Autodesk Inventor part; units mm, degrees
ref_plane "YZ Plane" through (0, 0, 0) normal (1, 0, 0) x (0, 1, 0)
ref_plane "XZ Plane" through (0, 0, 0) normal (0, 1, 0) x (-1, 0, 0)
ref_plane "XY Plane" through (0, 0, 0) normal (0, 0, 1) x (1, 0, 0)
sketch "Sketch1" plane through (0, 0, 0) normal (0, 1, 0) x (-1, 0, 0)
  line L0 (-10, 11.5) -> (10, 11.5)
  line L1 (10, 11.5) -> (10, -11.5)
  line L2 (10, -11.5) -> (-10, -11.5)
  line L3 (-10, -11.5) -> (-10, 11.5)
  line L4 (-10, 11.5) -> (10, -11.5) construction
  line L5 (10, 11.5) -> (-10, -11.5) construction
  point P0 (0, 0)
  dimension "d0" = 20
  dimension "d1" = 23
extrude "Extrusion2" add sketch "Sketch1" against normal blind 20
ref_plane "Work Plane1" through (-10, 0, 0) normal (0, 0, 1) x (1, 0, 0)
ref_plane "Work Plane2" through (0, -2, 0) normal (0, 1, 0) x (1, 0, 0)
sketch "Sketch11" plane through (0, -2, 0) normal (0, 1, 0) x (1, 0, 0)
  point P0 (0, 0)
sketch "Sketch12" plane through (10, 0, 11.5) normal (1, 0, 0) x (0, 0, -1)
  line L0 (23, -20) -> (0, -20)
  line L1 (0, -20) -> (0, 0)
  line L2 (0, 0) -> (23, 0)
  line L3 (23, 0) -> (23, -20)
  point P0 (11.5, 0)
  dimension "d41" = 23
  dimension "d42" = 20
extrude "Extrusion4" add sketch "Sketch12" along normal blind 22
sketch "Sketch13" plane through (32, 0, 11.5) normal (1, 0, 0) x (0, 0, -1)
  line L0 (23, 0) -> (23, -20)
  line L1 (23, -20) -> (3, -20)
  line L2 (3, -20) -> (3, 0)
  line L3 (3, 0) -> (23, 0)
  line L4 (23, 0) -> (23, -20)
  point P0 (11.5, 0)
  dimension "d45" = 20
extrude "Extrusion5" add sketch "Sketch13" along normal blind 120
sketch "Sketch26" plane through (32, -20, 8.5) normal (0, 0, 1) x (1, 0, 0)
  line L0 (8, 15) -> (23, 15)
  line L1 (23, 15) -> (23, 5)
  line L2 (23, 5) -> (8, 5)
  line L3 (8, 5) -> (8, 15)
  line L4 (0, 20) -> (120, 20)
  line L5 (0, 0) -> (120, 0)
  point P0 (-32, 20)
  dimension "d91" = 15
  dimension "d92" = 10
  dimension "d93" = 5
  dimension "d94" = 5
extrude "Extrusion12" cut sketch "Sketch26" against normal blind 15
sketch "Sketch28" plane through (10, 0, -11.5) normal (0, 0, -1) x (-1, 0, 0)
  line L0 (-22, 0) -> (-22, -20)
  line L1 (20, -20) -> (-142, -20)
  line L2 (-22, 0) -> (-142, 0)
  point P0 (10, 0)
  point P1 (-27, -17)
  point P2 (-46, -3)
  dimension "d101" = 19
  dimension "d102" = 5
  dimension "d103" = 3
  dimension "d104" = 3
hole "Hole3" at (56, -3, -11.5) at (37, -17, -11.5) direction (0, 0, 1) diameter 3.5 end through all counterbore diameter 5.5 counterbore depth 4
sketch "Sketch29" plane through (0, -20, 0) normal (0, -1, 0) x (1, 0, 0)
  line L0 (10, 11.5) -> (-10, 11.5)
  line L1 (10, -11.5) -> (10, 11.5)
  line L2 (-10, -11.5) -> (152, -11.5)
  line L3 (-10, 11.5) -> (-10, -11.5)
  point P0 (0, 0)
  point P1 (6.5, -8)
  point P2 (-6.5, 8)
  dimension "d112" = 3.5
  dimension "d113" = 3.5
  dimension "d128" = 3.5
  dimension "d129" = 3.5
hole "Hole4" at (-6.5, -20, 8) at (6.5, -20, -8) direction (0, 1, 0) diameter 3.7 end through all counterbore diameter 6 counterbore depth 4
sketch "Sketch38" plane through (0, -20, 0) normal (0, -1, 0) x (1, 0, 0)
  circle A0 centre (-6.5, 8) radius 3
  circle A1 centre (6.5, -8) radius 3
  circle A2 centre (-6.5, 8) radius 3
  circle A3 centre (6.5, -8) radius 3
  line L0 (-10, 11.5) -> (32, 11.5)
  line L1 (-10, 11.5) -> (-10, -11.5)
  line L2 (-10, -11.5) -> (152, -11.5)
  line L3 (152, 8.5) -> (152, -11.5)
  line L4 (32, 8.5) -> (152, 8.5)
  line L5 (32, 11.5) -> (32, 8.5)
  circle A4 centre (-6.5, 8) radius 3
  line L6 (-10, 11.5) -> (-10, -11.5)
  line L7 (-10, -11.5) -> (152, -11.5)
  line L8 (3.5, -11.5) -> (3.5, -8)
  circle A5 centre (6.5, -8) radius 3
  line L9 (9.5, -8) -> (9.5, -11.5)
  line L10 (-3.5, 11.5) -> (-3.5, 8)
  line L11 (-10, 11.5) -> (-10, -11.5)
  line L12 (-10, 5) -> (-6.5, 5)
  point P0 (0, 0)
extrude "Extrusion17" cut sketch "Sketch38" against normal up to surface (4 mm away) contours A0 L12 L1 L0 L10 | L8 A1 L9 L2
sketch "Sketch33" plane through (-10, -20, -11.5) normal (0, 0, -1) x (-1, 0, 0)
  circle A0 centre (-66, 17) radius 2.75
  circle A1 centre (-47, 3) radius 2.75
  line L0 (0, 20) -> (-162, 20)
  line L1 (0, 0) -> (-162, 0)
  circle A2 centre (-66, 17) radius 2.75
  line L2 (-63.25, 17) -> (-63.25, 20)
  line L3 (-68.749347, 16.940067) -> (-68.749347, 20)
  line L4 (-49.75, 3) -> (-49.75, 0)
  line L5 (-44.25, 3) -> (-44.25, 0)
  point P0 (-10, 20)
sketch "Sketch33 outline for Extrusion13" plane through (-10, -20, -11.5) normal (0, 0, -1) x (-1, 0, 0)
  arc A0 (-44.25, 3) -> (-49.75, 3) centre (-47, 3) cw
  line L0 (-44.25, 0) -> (-44.25, 3)
  line L1 (-49.75, 0) -> (-44.25, 0)
  line L2 (-49.75, 3) -> (-49.75, 0)
  arc A1 (-63.25, 17) -> (-68.749347, 17.059933) centre (-66, 17) ccw
  line L3 (-68.749347, 20) -> (-68.749347, 17.059933)
  line L4 (-63.25, 20) -> (-68.749347, 20)
  line L5 (-63.25, 17) -> (-63.25, 20)
extrude "Extrusion13" cut sketch "Sketch33 outline for Extrusion13" against normal up to surface (4 mm away)
sketch "Sketch34" plane through (32, 0, 11.5) normal (1, 0, 0) x (0, 0, -1)
  line L0 (3, -20) -> (3, 0)
  line L1 (3, 0) -> (0, 0)
  line L2 (0, 0) -> (0, -20)
  line L3 (0, -20) -> (3, -20)
  point P0 (11.5, 0)
extrude "ajustement" cut sketch "Sketch34" against normal blind 1
sketch "Sketch37" plane through (-10, -20, 11.5) normal (0, 0, 1) x (1, 0, 0)
  line L0 (20, 20) -> (20, 0) construction
  line L1 (0, 0) -> (41, 0) construction
  line L2 (20, 20) -> (40, 20) construction
  line L3 (50, 5) -> (50, 15) construction
  line L4 (50, 10) -> (20, 10) construction
  line L5 (50, 8.5) -> (17.5, 8.5)
  line L6 (17.5, 8.5) -> (14.5, 8.5)
  line L7 (14.5, 8.5) -> (14.5, 20)
  line L8 (41, 20) -> (0, 20)
  line L9 (50, 11.5) -> (17.5, 11.5)
  line L10 (17.5, 11.5) -> (17.5, 20)
  line L11 (17.5, 20) -> (14.5, 20)
  line L12 (50, 8.5) -> (50, 11.5)
  point P0 (10, 20)
  point P1 (20, 20)
  point P2 (0, 20)
  point P3 (17.5, 12)
  dimension "d137" = 90
  dimension "d138" = 2.5
  dimension "d139" = 1.5
  dimension "d140" = 1.5
  dimension "d141" = 3
ref_plane "Work Plane4" through (-10, -20, -4.5) normal (0, 0, 1) x (1, 0, 0)
extrude "Extrusion16" cut sketch "Sketch37" against normal up to surface (16 mm away)
fillet "Fillet1" radius 2 4 edges at (4.5, -11.5, 3.5) (7.5, -8.5, 3.5) (40, -11.5, 2) (40, -8.5, 2)
fillet "Fillet2" radius 3 1 edges at (55, -5, 1)
sketch "Sketch39" plane through (152, -20, 8.5) normal (0, 0, 1) x (1, 0, 0)
  arc A0 (-97, 12) -> (-100, 15) centre (-100, 12) ccw
  line L0 (-112, 15) -> (-100, 15)
  line L1 (-112, 5) -> (-112, 15)
  line L2 (-97, 5) -> (-112, 5)
  line L3 (-97, 12) -> (-97, 5)
  line L4 (-121, 11.5) -> (-121, 20)
  circle A1 centre (-115, 3) radius 1.75
  line L5 (-121, 0) -> (-121, 8.5)
  point P0 (-152, 20)
  point P1 (-104.5, 10)
  dimension "d149" = 16.5
  dimension "d150" = 6
ref_plane "Work Plane5" through (69, 0, 11.5) normal (1, 0, 0) x (0, 0, -1)
sketch "Sketch41" plane through (152, 0, 11.5) normal (1, 0, 0) x (0, 0, -1)
  line L0 (3, -20) -> (23, -20)
  line L1 (23, -20) -> (23, 0)
  line L2 (23, 0) -> (3, 0)
  line L3 (3, 0) -> (3, -20)
  line L4 (3, -20) -> (23, -20)
  line L5 (5, -20) -> (3, -18)
  line L6 (21, -20) -> (23, -18)
  line L7 (23, -2) -> (21, 0)
  line L8 (23, 0) -> (3, 0)
  line L9 (5, 0) -> (3, -2)
  point P0 (11.5, 0)
  dimension "d152" = 2
  dimension "d153" = 2
  dimension "d154" = 2
  dimension "d155" = 2
  dimension "d156" = 2
  dimension "d157" = 2
  dimension "d158" = 2
  dimension "d159" = 2
extrude "Extrusion18" cut sketch "Sketch41" against normal up to surface (83 mm away) contours L3 L5 L0 | L6 L1 L0 | L3 L2 L9 | L7 L2 L1
equation "\"d93\" = d94"
equation "\"d140\" = d139"
equation "\"d153\" = d152"
equation "\"d154\" = d152"
equation "\"d155\" = d152"
equation "\"d156\" = d152"
equation "\"d158\" = d152"
properties part number "bas_de_fourche_gros_bloc"
Geometry: final body of the model. Coordinates: model frame, mm. A direction names the side the tool comes from. Coordinates: 2 decimals unless noted, no trailing zeros. Order: outer loops, then holes, each group sorted by start corner. A loop starts at its lowest first (then second) coordinate and runs counter-clockwise, first axis right, second up. Notation, with made-up numbers: (88, 11.5) -> (100, 11.5) arc R20 cw to (100, 35.5) -> close; hole circle Ø2 at (56.25, 72). An arc over 180 degrees is marked (long way). Answer in a Markdown table with one row per item.
Item 1: Contact query for flat-ended pins moving along their axis: P1, Ø4.5, axis at x = -6.5, z = 8, coming from the -Y side; P2, Ø5, axis at x = 49.5, y = -8, coming from the +Z side; P3, Ø2, axis at x = 56, y = -3, coming from the -Z side; P4, Ø10, axis at x = 66.5, y = -10, coming from the +Z side. Output: stop coordinate, or through.
Return value:
| item | result |
|---|---|
| P1 | stops at y = -16 |
| P2 | stops at z = -6.5 |
| P3 | passes through |
| P4 | stops at z = 8.5 |
Item 2: Draft query along Y for faces 6 (the flat face through (70, -20, 0)), 7 (the flat face through (53.25, -2, -10)), 8 (the cylindrical face through (38.06, -18.39, 0.61)). Return one class per face: released by +Y, released by -Y, zero draft, split by the parting line, or undercut.
Return value:
| item | result |
|---|---|
| face 6 | released by -Y |
| face 7 | zero draft |
| face 8 | undercut |
Item 3: Section B-B on z = 2.25. Output: boundary loops of the cut face in (x, y).
Return value:
| item | result |
|---|---|
| outline | (-10, -20) -> (152, -20) -> (152, 0) -> (7.5, 0) -> (7.5, -6.5) arc R2 ccw to (9.5, -8.5) -> (38, -8.5) arc R2 ccw to (40, -6.5) -> (40, -5) -> (52, -5) arc R3 cw to (55, -8) -> (55, -15) -> (40, -15) -> (40, -13.5) arc R2 ccw to (38, -11.5) -> (6.5, -11.5) arc R2 cw to (4.5, -9.5) -> (4.5, 0) -> (-10, 0) -> close; hole circle Ø3.5 at (37, -17); hole circle Ø3.5 at (56, -3) |
Item 4: Section A-A on x = 29.5. Output: boundary loops of the cut face in (y, z), plus the area to 3 significant figures.
Return value:
| item | result |
|---|---|
| outline | (-20, -11.5) -> (0, -11.5) -> (0, 11.5) -> (-8.5, 11.5) -> (-8.5, -4.5) -> (-11.5, -4.5) -> (-11.5, 11.5) -> (-20, 11.5) -> close |
| area | 412 mm² |
Item 5: Access query for faces 1 (the flat face through (31, -16, 10)), 2 (the flat face through (4.5, -5, 4)), 3 (the flat face through (58.749, -1, -10)), 4 (the flat face through (20, -9, -4.5)), 5 (the flat face through (37, -19, -7.5)). Directions: +Z, -Z, +X, -X, +Y, -Y. A direction counts if a zero-diameter tool reaches every point of the face in a straight line with its end or side. Return the directions, or none.
Return value:
| item | result |
|---|---|
| face 1 | +Z, +X, +Y, -Y |
| face 2 | +Z, +Y |
| face 3 | -Z, +Y |
| face 4 | +Z |
| face 5 | -Z, -Y |
Item 6: Ray query, L1, parallel to Y at x = 37, z = 4; L2, parallel to X at y = -9, z = 8; L3, parallel to Z at x = 6.5, y = -3.5. Return the intervals inside material, ascending.
Return value:
| item | result |
|---|---|
| L1 | y = -20 to -18.75, -15.25 to -11.5, -8.5 to 0 |
| L2 | x = -10 to -8.35, -4.65 to 4.5, 55 to 152 |
| L3 | z = -11.5 to -9.85, -6.15 to -4.5 |
